Verification items for the finished model (mm, model axes). Give positions to 0.01 mm unless a question says otherwise; leave off trailing zeros. Write each loop counter-clockwise with the first axis right and the second up, starting at its lowest first coordinate (ties: lowest second). Pieces come first, ordered by that corner, then holes.
from build123d import *

# Parameters (mm, degrees)
SKETCH1_R           = 25.654
SKETCH1_R_2         = 21.717
BOSS_EXTRUDE1_DEPTH = 279.4
CUT_EXTRUDE1_START  = 19.05
CUT_EXTRUDE1_DEPTH  = 12.7
LPATTERN1_COUNT     = 13
LPATTERN1_PITCH     = 13.462


with BuildPart() as part:
    # Sketch1 → Boss-Extrude1 (new body)
    with BuildSketch(Plane(origin=(0, 0, 0), x_dir=(1, 0, 0), z_dir=(0, 1, 0))):
        Circle(SKETCH1_R)
        Circle(SKETCH1_R_2, mode=Mode.SUBTRACT)
    extrude(amount=BOSS_EXTRUDE1_DEPTH)

    # Sketch2 → Cut-Extrude1 (cut)
    with BuildSketch(Plane.XY.offset(CUT_EXTRUDE1_START)):
        Polygon((-29.021596045, 224.724403955), (-25.654, 221.356807909), (29.021596045, 276.032403955), (25.654, 279.4), align=None)
    cut_extrude1 = extrude(amount=CUT_EXTRUDE1_DEPTH, mode=Mode.SUBTRACT)

    # LPattern1: Cut-Extrude1 ×13
    with Locations(*[(0, -i * LPATTERN1_PITCH, 0) for i in range(1, LPATTERN1_COUNT)]):
        add(cut_extrude1, mode=Mode.SUBTRACT)


solid = part.part
Item 1: Sectioned sample at B-B on z = 0. Record the cut outline in (x, y), then the cut area to 3 significant figures.
Answer key:
outline: (-25.65, 0) - (-21.72, 0) - (-21.72, 279.4) - (-25.65, 279.4) - close; (21.72, 0) - (25.65, 0) - (25.65, 279.4) - (21.72, 279.4) - close
area: 2,200 mm2
Item 2: Depth check by flat-ended pin: pin 1 (7.5 mm diameter, centred on x = -14, y = 221, fed in from +Z); pin 2 (2 mm diameter, centred on x = -12, y = 193.5, fed in from +Z); pin 3 (7.5 mm diameter, centred on x = -14.5, y = 154.5, fed in from +Z); pin 4 (8 mm diameter, centred on x = 11.5, z = 8.5, fed in from +Y). Enter the tip coordinate at first touch or a pass-through.
Answer key:
pin 1: stops at z = 23.52
pin 2: stops at z = 23.18
pin 3: stops at z = 23.29
pin 4: passes through
Item 3: Scan lines: line 1 along Z through (x, y) = (0, 201); line 2 along Z through (x, y) = (1, 169). Record each from-to range of solid material in increasing order.
Answer key:
line 1: z = -25.65 to -21.72, 21.72 to 25.65
line 2: z = -25.63 to -21.69
Item 4: Sectioned sample at C-C on x = 0. State how many separate pieces and enclosed holes the cut face has, then the cut area to 3 significant figures.
Answer key:
separate pieces: 15
enclosed holes: 0
area: 1,860 mm2
Item 5: Sectioned sample at A-A on z = 11. Record the cut outline in (x, y), then the cut area to 3 significant figures.
Answer key:
outline: (-23.18, 0) - (-18.73, 0) - (-18.73, 279.4) - (-23.18, 279.4) - close; (18.73, 0) - (23.18, 0) - (23.18, 279.4) - (18.73, 279.4) - close
area: 2,490 mm2
